Input: dimensioned drawing with shaded views. Units: mm. Origin: part minimum x, y, z. A direction names the side the tool comes from. Coordinates: 2 decimals unless noted, no trailing zeros. Loops run counter-clockwise (first coordinate to the right, second up) from the corner with the lowest first, then second, coordinate; pieces in that order, holes last.
Item 1: Ray query, line 1 along Z through (x, y) = (3, 4) (1 decimal); line 2 along Y through (x, z) = (5.25, 4.5); line 3 along X through (y, z) = (5.25, 9.25) (1 decimal). Return the intervals inside material, ascending.
Item 2: Section B-B on y = 5.5. Give the number of separate pieces and of enclosed holes in the cut face.
Item 3: Section C-C on x = 7.5. Return loops of the section in (y, z).
Item 4: Contact query for flat-ended pins moving along their axis: P1, Ø1.5, axis at x = 4, y = 9.5, coming from the -Z side; P2, Ø3, axis at y = 3, z = 5.5, coming from the -X side; P3, Ø4, axis at x = 7, z = 5, coming from the +Y side. Output: stop coordinate, or through.
Item 5: Pull-direction query (Z, two-part tool) for the marked faces 1, 2 and 3; classes: released by +Z, released by -Z, zero draft, split by the parting line, or undercut.
Item 6: Section A-A on x = 3. Return loops of the section in (y, z), and give its area (3 significant figures).
Item 7: Section D-D on z = 9. Return loops of the section in (x, y) (1 decimal).
Item 8: Reachability of the marked faces 4, 5 and 6 from +Z, -Z, +X, -X, +Y, -Y: full face, straight path, thin tool, end or side. Return the list, or none.
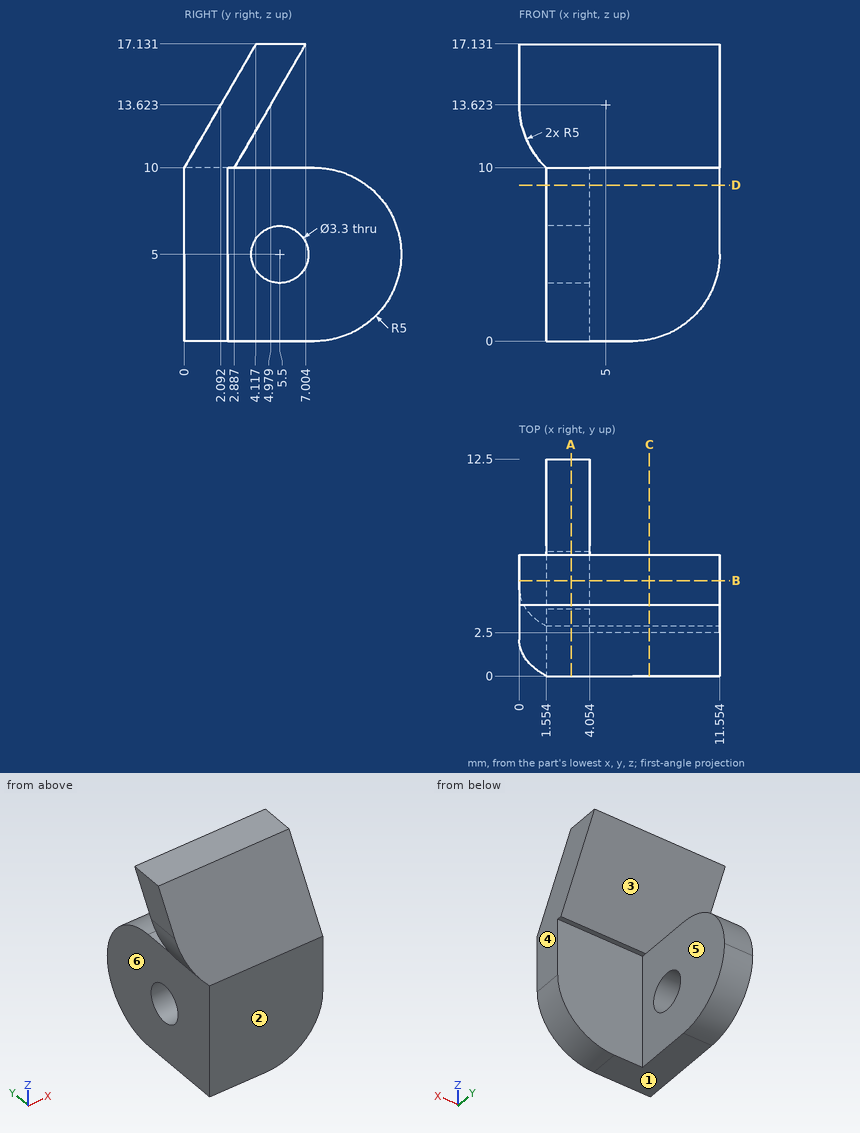
Results found:
1. line 1: z = 0 to 4.3, 5.7 to 10, 11.9 to 16.9
1. line 2: y = 0 to 2.5
1. line 3: x = 1.6 to 4.1
2. separate pieces: 3
2. enclosed holes: 0
3. outline: (0, 0.09) - (2.5, 0.09) - (2.5, 10) - (2.89, 10) - (7, 17.13) - (4.12, 17.13) - (0, 10) - close
4. P1: stops at z = 0.16
4. P2: stops at x = 1.55
4. P3: stops at y = 2.5
5. face 1: released by -Z
5. face 2: zero draft
5. face 3: undercut
6. outline: (0, 0) - (7.5, 0) arc R5 ccw to (7.5, 10) - (2.89, 10) - (7, 17.13) - (4.12, 17.13) - (0, 10) - close; hole circle Ø3.3 at (5.5, 5)
6. area: 126 mm2
7. outline: (1.6, 0) - (11.6, 0) - (11.6, 2.5) - (4.1, 2.5) - (4.1, 10.5) - (1.6, 10.5) - close
8. face 4: +Z, -Z, +X, +Y, -Y
8. face 5: -Z, +X, +Y
8. face 6: -Z, -X, +Y, -Y
